Answer from the drawing. Dimensions are ordinates in mm from the lowest x, y and z of the part. Give positions to 0.01 mm unless a question says otherwise; leave off trailing zeros. Write each loop counter-clockwise with the first axis right and the second up, starting at its lowest first coordinate (ties: lowest second). Pieces come first, ordered by that corner, then holes.
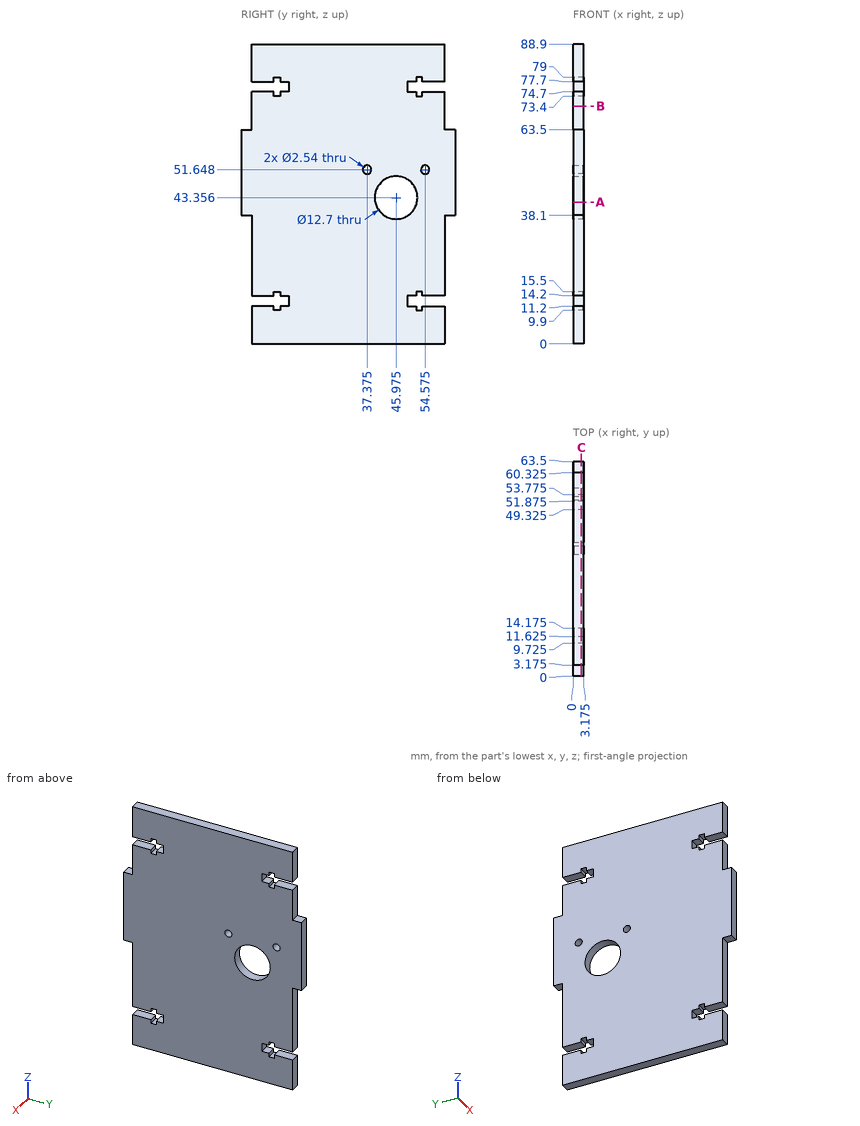
Item 1: Consider probe 1 along Z at (x, y) = (0.6, 57.5); probe 2 along Z at (x, y) = (2.9, 10); probe 3 along Y at (x, z) = (0.95, 74.5) (1 decimal). Determine where each line is inside the solid, lowest interval first.
Conclusion:
probe 1: z = 0 to 11.2, 14.2 to 74.7, 77.7 to 88.9
probe 2: z = 0 to 9.9, 15.5 to 73.4, 79 to 88.9
probe 3: y = 3.2 to 9.7, 11.6 to 51.9, 53.8 to 60.3
Item 2: A cutting plane is placed at B-B, the plane z = 70.5. Give the vertices of the cut face in (x, y) (1 decimal).
Conclusion:
outline: (0, 3.2) - (3.2, 3.2) - (3.2, 60.3) - (0, 60.3) - close
Item 3: A cutting plane is placed at A-A, the plane z = 42. Give the vertices of the cut face in (x, y) (1 decimal), plus the area to 3 significant figures.
Conclusion:
outline: (0, 0) - (3.2, 0) - (3.2, 39.8) - (0, 39.8) - close; (0, 52.2) - (3.2, 52.2) - (3.2, 63.5) - (0, 63.5) - close
area: 162 mm2
Item 4: Each of these flat-tipped pins is pushed along its axis until it touches: P1, Ø1, axis at x = 1, z = 15, coming from the -Y side (3 decimals); P2, Ø1.4, axis at x = 1.5, z = 15, coming from the +Y side (3 decimals). Where does it stop, or does it pass through?
Conclusion:
P1: stops at y = 3.175
P2: stops at y = 60.325
Item 5: A cutting plane is placed at C-C, the plane x = 2.45. Count the separate pieces of the cut face and the enclosed holes in it, plus the area to 3 significant figures.
Conclusion:
separate pieces: 1
enclosed holes: 3
area: 4,950 mm2
